Read the model definition and answer for the solid it produces. Units are mm, in the model's axes. Face numbers are marked on the shaded views. A direction names the side the tool comes from. Coordinates: 2 decimals unless noted, no trailing zeros. Order: outer loops, then holes, each group sorted by start corner. A loop starts at its lowest first (then second) coordinate and runs counter-clockwise, first axis right, second up. Notation, with made-up numbers: (6, 60) -> (59, 60) arc R19 ccw to (59, 65) -> close; hole circle Ø7 at (-13.5, 56). An arc over 180 degrees is marked (long way). Answer as a JSON object with one key per item and string values. Group by question number.
1) Section D-D on x = 15.5 is taken. Determine the outline of the cut face in (y, z) (3 decimals), and give its area (3 significant figures).
2) Determine the mould class of the marked faces 1, 2, 3 and 4 for opening direction X: released by +X, released by -X, zero draft, split by the parting line, or undercut.
3) Given pin 1 (5 mm diameter, centred on x = 5, y = 0.5, fed in from +Z); pin 2 (12 mm diameter, centred on x = 9.5, z = 1.5, fed in from -Y); pin 3 (5 mm diameter, centred on x = 15, y = 4.5, fed in from -Z), each flat-ended and moving along its own axis, determine where each tip first touches the part or whether it passes through.
4) Consider L1, parallel to Y at x = 6.5, z = 0 (3 decimals); L2, parallel to X at y = 1.25, z = 3.5; L3, parallel to X at y = -3.5, z = -7. Determine where each line is inside the solid, lowest interval first.
5) Section A-A on x = 24 is taken. Determine the outline of the cut face in (y, z) (3 decimals).
6) A tool of negligible diameter and unlimited length cuts with its end or side. For the marked faces 5, 6 and 7, from which of +Z, -Z, +X, -X, +Y, -Y can it reach the whole face along a straight path? Write none if from no direction.
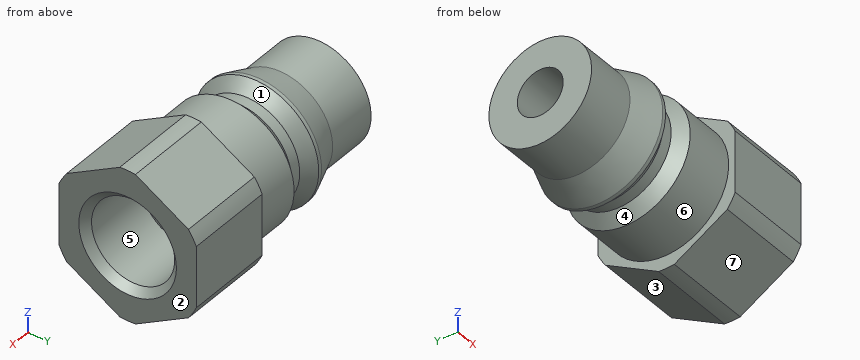
from build123d import *

# Parameters (mm, degrees)
CUT_EXTRUDE1_DEPTH       = 38.964720465
SCHIZZO1_R               = 5.75
TAGLIO_ESTRUSIONE1_DEPTH = 10
SMUSSO1_SIZE             = 1


with BuildPart() as part:
    # Sketch1 → Revolve1 (revolve)
    with BuildSketch(Plane.XY, mode=Mode.PRIVATE) as revolve1_sk:
        Polygon((0, -7.1), (7, -7.1), (11, -8.6), (11.5, -8.6), (13, -7.1), (14.5, -7.1), (16, -8.6), (23, -8.6), (23, -10.4), (35, -10.4), (35, -3.175), (0, -3.175), align=None)
    revolve(revolve1_sk.sketch.rotate(Axis((0, 0, 0), (1, 0, 0)), 270), axis=Axis((0, 0, 0), (1, 0, 0)))

    # Sketch2 → Cut-Extrude1 (cut, through all)
    with BuildSketch(Plane(origin=(35, 0, 0), x_dir=(0, 0, -1), z_dir=(1, 0, 0))):
        with BuildLine():
            Line((-10.343251733, 1.084962483), (-6.111230939, 8.415037517))
            ThreePointArc((-6.111230939, 8.415037517), (-9.006664199, 5.2), (-10.343251733, 1.084962483))
        make_face()
        with BuildLine():
            ThreePointArc((4.232020794, 9.5), (0, 10.4), (-4.232020794, 9.5))
            Line((-4.232020794, 9.5), (4.232020794, 9.5))
        make_face()
        with BuildLine():
            Line((-6.111230939, -8.415037517), (-10.343251733, -1.084962483))
            ThreePointArc((-10.343251733, -1.084962483), (-9.006664199, -5.2), (-6.111230939, -8.415037517))
        make_face()
        with BuildLine():
            ThreePointArc((10.343251733, 1.084962483), (9.006664199, 5.2), (6.111230939, 8.415037517))
            Line((6.111230939, 8.415037517), (10.343251733, 1.084962483))
        make_face()
        with BuildLine():
            Line((4.232020794, -9.5), (-4.232020794, -9.5))
            ThreePointArc((-4.232020794, -9.5), (0, -10.4), (4.232020794, -9.5))
        make_face()
        with BuildLine():
            ThreePointArc((6.111230939, -8.415037517), (9.006664199, -5.2), (10.343251733, -1.084962483))
            Line((10.343251733, -1.084962483), (6.111230939, -8.415037517))
        make_face()
    extrude(amount=-CUT_EXTRUDE1_DEPTH, mode=Mode.SUBTRACT)

    # Schizzo1 → Taglio-Estrusione1 (cut)
    with BuildSketch(Plane(origin=(35, 0, 0), x_dir=(0, 0, -1), z_dir=(1, 0, 0))):
        Circle(SCHIZZO1_R)
    extrude(amount=-TAGLIO_ESTRUSIONE1_DEPTH, mode=Mode.SUBTRACT)

    # Smusso1
    smusso1_edges = [part.edges().sort_by_distance(p)[0] for p in [
        (35, 0, 5.75),
    ]]
    chamfer(smusso1_edges, length=SMUSSO1_SIZE)


solid = part.part
Worked answers:
{
 "1": {"outline": "circle Ø16.2 at (0, 0); hole circle Ø6.35 at (0, 0)", "area": "174 mm²"},
 "2": {"face 1": "undercut", "face 2": "released by +X", "face 3": "zero draft", "face 4": "undercut"},
 "3": {"pin 1": "stops at z = 7.28", "pin 2": "stops at y = -8.6", "pin 3": "stops at z = -8.31"},
 "4": {"L1": "y = -7.1 to -3.175, 3.175 to 7.1", "L2": "x = 0 to 25", "L3": "x = 8.94 to 12.27, 15.23 to 35"},
 "5": {"outline": "(-9.5, -4.232) arc R10.4 ccw to (-8.415, -6.111) -> (-1.085, -10.343) arc R10.4 ccw to (1.085, -10.343) -> (8.415, -6.111) arc R10.4 ccw to (9.5, -4.232) -> (9.5, 4.232) arc R10.4 ccw to (8.415, 6.111) -> (1.085, 10.343) arc R10.4 ccw to (-1.085, 10.343) -> (-8.415, 6.111) arc R10.4 ccw to (-9.5, 4.232) -> close; hole circle Ø6.35 at (0, 0)"},
 "6": {"face 5": "+X", "face 6": "-X", "face 7": "-Z, +X, -X, -Y"}
}
